Can you work these out from the model? Positions are in its coordinate system, mm. A direction names the side the tool comes from. Round coordinates to 2 decimals unless told otherwise and drop trailing zeros. Loops run counter-clockwise (first coordinate to the right, second up) from the corner with the lowest first, then second, coordinate; pieces in that order, holes last.
(1) I want a section at A-A on z = -1. Write out the boundary of the cut face in (x, y), plus the area to 3 significant figures.
(2) I want a section at C-C on x = 37. Write out the boundary of the cut face in (y, z).
(3) If I drill on line 1 along Z through (x, y) = (30, 4); line 2 along Y through (x, z) = (19.5, 6.5); line 3 along X through (y, z) = (4.75, 0), over which ranges is the centre line in solid material (lowest first)?
(4) I want a section at B-B on y = 42.5. Write out the boundary of the cut face in (x, z).
(5) Thinking about a two-plate mould opening in Y: for faces 1 (the face through (26.99, 44.99, -17.15)), 2 (the face through (21, 0, -5)), 3 (the face through (13.01, 12.85, -0.28)), 4 (the face through (42, 10, 0)), which applies, released by +Y, released by -Y, zero draft, split by the parting line, or undercut?
(6) Will these pins go through, and if not, where does the flat tip stop? pin 1 Ø11 at (y, z) = (42.5, -3) entering from +X; pin 2 Ø6 at (y, z) = (33.5, -5.5) entering from +X.
(7) Which directions (+Z, -Z, +X, -X, +Y, -Y) give clear straight access to the entire face, cutting with the end or side of a thin tool? Please do faces 5 (the face through (30, 45, 0)), 6 (the face through (10, 30, 0)), 7 (the face through (39.76, 5.07, 2.17)), 8 (the face through (27.15, 44.99, 16.99)).
Autodesk Inventor part; units mm, degrees
ref_plane "YZ Plane" through (0, 0, 0) normal (1, 0, 0) x (0, 1, 0)
ref_plane "XZ Plane" through (0, 0, 0) normal (0, 1, 0) x (-1, 0, 0)
ref_plane "XY Plane" through (0, 0, 0) normal (0, 0, 1) x (1, 0, 0)
sketch "Sketch1" plane through (0, 0, 0) normal (0, 0, 1) x (1, 0, 0)
  line L0 (0, 60.4862) -> (0, -12.4973)
  line L1 (-12.4853, 0) -> (60.4142, 0)
  line L2 (0, 50.06) -> (30, 50.06)
  line L3 (30, 50.06) -> (30, 40.06)
  line L4 (30, 40.06) -> (10, 40.06)
  line L5 (0, 40.06) -> (0, 50.06)
  line L6 (10, 0) -> (50, 0)
  line L7 (50, 0) -> (50, 10)
  line L8 (50, 10) -> (20, 10)
  line L9 (0, 10) -> (0, 10)
  line L10 (10, 40.06) -> (10, 20)
  line L11 (0, 10) -> (0, 40.06)
  arc A0 (0, 10) -> (10, 0) centre (10, 10) ccw
  arc A1 (10, 20) -> (20, 10) centre (20, 20) ccw
  point P0 (0, 0)
  dimension "d0" = 30
  dimension "d2" = 50
  dimension "d3" = 10
  dimension "d5" = 10
  dimension "d6" = 10
extrude "Extrusion1" add sketch "Sketch1" along normal mid plane 40 contours L2 L3 L4 L10 A1 L8 L7 L1 A0 L0
fillet "Fillet1" radius 20 2 edges at (50, 5, 20) (50, 5, -20)
fillet "Fillet2" radius 10 2 edges at (30, 45.06, 20) (30, 45.06, -20)
sketch "Sketch2" plane through (10, 0, -20) normal (0, -1, 0) x (1, 0, 0)
  arc A0 (20, 0) -> (20, 40) centre (20, 20) ccw
  point P0 (-10, 20)
hole "Hole1" at (30, 0, 0) direction (0, 1, 0) diameter 20 depth 10
properties part number "Exercise_3"
Filled sheet:
1. outline: (0, 10) arc R10 ccw to (10, 0) - (20.05, 0) - (20.05, 10) - (20, 10) arc R10 cw to (10, 20) - (10, 40.06) - (30, 40.06) - (30, 50.06) - (0, 50.06) - close; (39.95, 0) - (49.97, 0) - (49.97, 10) - (39.95, 10) - close
1. area: 901 mm2
2. outline: (0, -18.74) - (10, -18.74) - (10, -7.14) - (0, -7.14) - close; (0, 7.14) - (10, 7.14) - (10, 18.74) - (0, 18.74) - close
3. line 1: z = -20 to -10, 10 to 20
3. line 2: y = 0 to 10.01, 40.06 to 50.06
3. line 3: x = 1.49 to 20, 40 to 50
4. outline: (0, -20) - (20, -20) arc R10 ccw to (30, -10) - (30, 10) arc R10 ccw to (20, 20) - (0, 20) - close
5. face 1: zero draft
5. face 2: released by -Y
5. face 3: undercut
5. face 4: undercut
6. pin 1: stops at x = 30
6. pin 2: stops at x = 10
7. face 5: +Z, -Z, +X, +Y, -Y
7. face 6: +Z, -Z, +X
7. face 7: -Y
7. face 8: +Z, +X, +Y
